Geometry check sheet. Reference: the model listing, model coordinates, mm. A direction names the side the tool comes from. Give positions to 0.01 mm unless a question says otherwise; leave off trailing zeros. Write each loop counter-clockwise with the first axis right and the second up, starting at its lowest first coordinate (ties: lowest second). Pieces come first, ordered by that corner, then holes. Notation, with made-up numbers: (-7.5, 1.5) -> (29.5, 1.5) arc R26 ccw to (29.5, 38.5) -> close; hole circle Ø9 at (71.25, 83). An arc over 180 degrees is marked (long way). Use a Markdown table: item, result. Add a question column.
from build123d import *

# Parameters (mm, degrees)
SKETCH_2_W          = 33.1
SKETCH_2_H          = 9.1
EXTRUDE_1_DEPTH     = 9
SKETCH_3_W          = 30.9
SKETCH_3_H          = 6.9
CUT_EXTRUDE_1_DEPTH = 7.5
SKETCH_4_W          = 4.5
SKETCH_4_H          = 1.1
CUT_EXTRUDE_2_DEPTH = 7.5


with BuildPart() as part:
    # Эскиз2 → Бобышка-Вытянуть1 (new body)
    with BuildSketch(Plane.XY):
        Rectangle(SKETCH_2_W, SKETCH_2_H)
    extrude(amount=EXTRUDE_1_DEPTH)

    # Эскиз3 → Вырез-Вытянуть1 (cut)
    with BuildSketch(Plane.XY.offset(9)):
        Rectangle(SKETCH_3_W, SKETCH_3_H)
    extrude(amount=-CUT_EXTRUDE_1_DEPTH, mode=Mode.SUBTRACT)

    # Эскиз4 → Вырез-Вытянуть2 (cut)
    with BuildSketch(Plane.XY.offset(9)):
        with Locations((0, 4)):
            Rectangle(SKETCH_4_W, SKETCH_4_H)
    extrude(amount=-CUT_EXTRUDE_2_DEPTH, mode=Mode.SUBTRACT)


solid = part.part
1) Material ranges on probe 1 along Y at (x, z) = (12, 6.25); probe 2 along X at (y, z) = (-0.5, 1.75); probe 3 along X at (y, z) = (4, 2.5), recorded low to high. Write a range as [from, to].
2) Tool access check on faces 4 (the face through (-2.25, 4, 5)), 5 (the face through (9, 3.45, 5)), 6 (the face through (0, -4.55, 4)). Record the directions out of +Z, -Z, +X, -X, +Y, -Y that give a thin tool (end or side, any length) a straight path to the whole face; none if there is none.
3) Draft check along X on faces 1 (the face through (16.55, 0, 4)), 2 (the face through (0, 4.55, 1)), 3 (the face through (15.45, 0, 5)). Enter one of: +X half, -X half, draft (parallel to the pull), parting line (faces both ways), or undercut.
4) Sectioned sample at C-C, the plane x = -12. Enter the section's corners in (y, z), and give its area (4 significant figures).
5) Gauge pin test, flat end, axial feed: P1, Ø1.5, axis at x = -8, y = 2.5, coming from the +Z side. Record the tip position at first contact, or that the pin passes through.
6) Sectioned sample at B-B, the plane z = 2.75. Enter the section's corners in (x, y).
7) Sectioned sample at A-A, the plane y = 3.75. Enter the section's corners in (x, z).
Check values:
| question | item | result |
|---|---|---|
| 1 | probe 1 | [-4.55, -3.45], [3.45, 4.55] |
| 1 | probe 2 | [-16.55, -15.45], [15.45, 16.55] |
| 1 | probe 3 | [-16.55, -2.25], [2.25, 16.55] |
| 2 | face 4 | +Z, +Y |
| 2 | face 5 | +Z |
| 2 | face 6 | +Z, -Z, +X, -X, -Y |
| 3 | face 1 | +X half |
| 3 | face 2 | draft |
| 3 | face 3 | undercut |
| 4 | outline | (-4.55, 0) -> (4.55, 0) -> (4.55, 9) -> (3.45, 9) -> (3.45, 1.5) -> (-3.45, 1.5) -> (-3.45, 9) -> (-4.55, 9) -> close |
| 4 | area | 30.15 mm² |
| 5 | P1 | z = 1.5 |
| 6 | outline | (-16.55, -4.55) -> (16.55, -4.55) -> (16.55, 4.55) -> (2.25, 4.55) -> (2.25, 3.45) -> (15.45, 3.45) -> (15.45, -3.45) -> (-15.45, -3.45) -> (-15.45, 3.45) -> (-2.25, 3.45) -> (-2.25, 4.55) -> (-16.55, 4.55) -> close |
| 7 | outline | (-16.55, 0) -> (16.55, 0) -> (16.55, 9) -> (2.25, 9) -> (2.25, 1.5) -> (-2.25, 1.5) -> (-2.25, 9) -> (-16.55, 9) -> close |
